Print and shaded views of the part. All mm, measured from the part's lowest x, y and z. A direction names the side the tool comes from. Give positions to 0.01 mm unless a question says otherwise; leave off trailing zeros. Write each loop counter-clockwise with the first axis right and the second up, starting at its lowest first coordinate (ties: lowest second). Pieces come first, ordered by that corner, then holes.
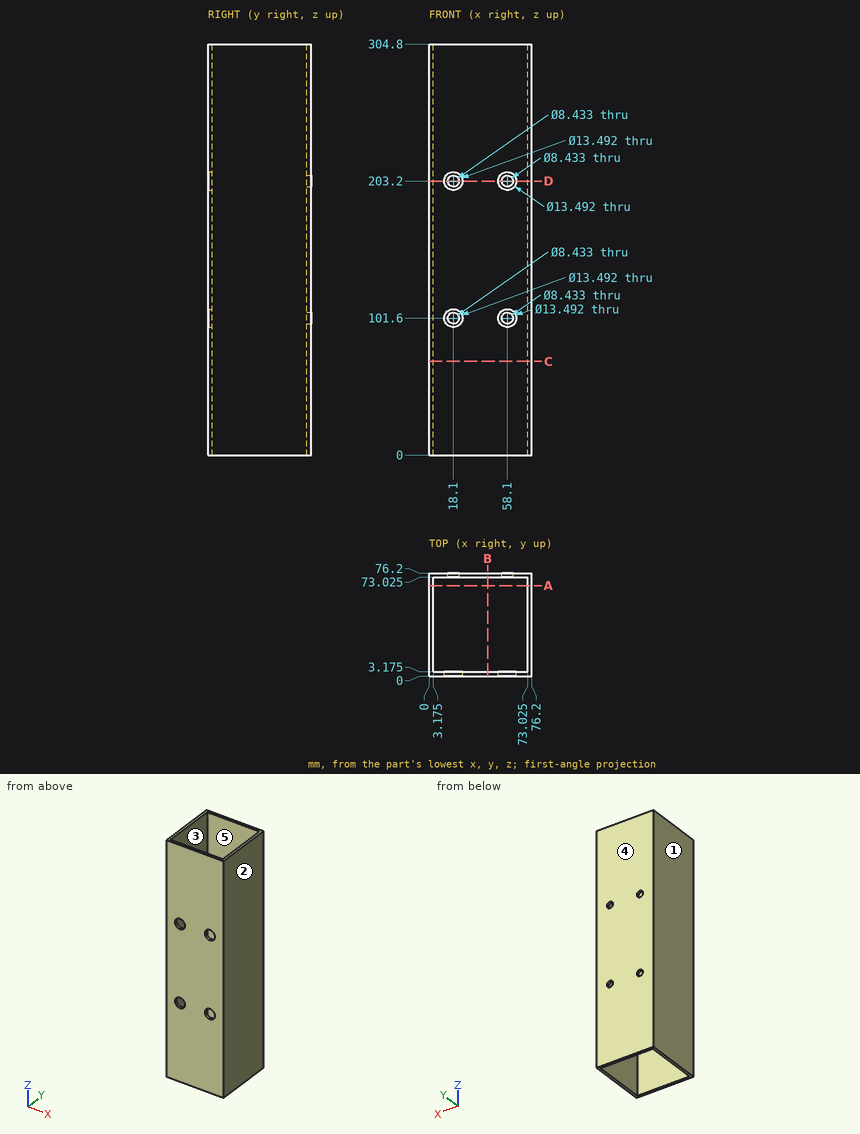
1. Saw through at D-D on z = 203.2. Give the cut face in (x, y) (1 decimal).
2. Drop a flat-ended pin along its axis: pin 1 (11 mm diameter, centred on x = 18.1, z = 101.6, fed in from -Y) (1 decimal). Give the stop position or say it passes through.
3. Saw through at A-A on y = 67. Give the cut face in (x, z) (1 decimal).
4. Saw through at C-C on z = 69.5. Give the cut face in (x, y) (1 decimal).
5. Drill centre lines: line 1 along X through (y, z) = (75, 101); line 2 along Z through (x, y) = (18.1, 74.3); line 3 along Z through (x, y) = (18.1, 0.9). Where is each one in solid material? Low to high.
6. Mould opens along X. For the marked faces 1, 2 and 3 say: pulls with the +X half, pulls with the -X half, needs draft (parallel to the pull), parting line crosses it, or undercut.
7. 3-axis set-ups, long thin cutter, end or side, ignore diameter. For the marked faces 4 and 5: which of +Z, -Z, +X, -X, +Y, -Y reach the whole face in a straight line?
Outcome:
1. outline: (0, 0) - (11.4, 0) - (11.4, 3.2) - (3.2, 3.2) - (3.2, 73) - (13.9, 73) - (13.9, 76.2) - (0, 76.2) - close; (22.3, 73) - (53.9, 73) - (53.9, 76.2) - (22.3, 76.2) - close; (24.8, 0) - (51.4, 0) - (51.4, 3.2) - (24.8, 3.2) - close; (62.3, 73) - (73, 73) - (73, 3.2) - (64.8, 3.2) - (64.8, 0) - (76.2, 0) - (76.2, 76.2) - (62.3, 76.2) - close
2. pin 1: stops at y = 73
3. outline: (0, 0) - (3.2, 0) - (3.2, 304.8) - (0, 304.8) - close; (73, 0) - (76.2, 0) - (76.2, 304.8) - (73, 304.8) - close
4. outline: (0, 0) - (76.2, 0) - (76.2, 76.2) - (0, 76.2) - close; hole (3.2, 3.2) - (73, 3.2) - (73, 73) - (3.2, 73) - close
5. line 1: x = 0 to 13.93, 22.27 to 53.93, 62.27 to 76.2
5. line 2: z = 0 to 97.38, 105.82 to 198.98, 207.42 to 304.8
5. line 3: z = 0 to 94.85, 108.35 to 196.45, 209.95 to 304.8
6. face 1: pulls with the -X half
6. face 2: pulls with the +X half
6. face 3: undercut
7. face 4: +Z, -Z, +X, -X, +Y
7. face 5: +Z, -Z
